Part model, mm, in its own coordinate system. A direction names the side the tool comes from. Round coordinates to 2 decimals unless told otherwise and drop trailing zeros. Loops run counter-clockwise (first coordinate to the right, second up) from the corner with the lowest first, then second, coordinate; pieces in that order, holes last. Notation, with made-up numbers: M 9.5,55.5 L 50.5,55.5 A35 cw 50.5,93.5 Z; hole C 1.5,23 d11. An arc over 180 degrees is marked long. Write each question's results on one line, items separated by ' | '.
from build123d import *

# Parameters (mm, degrees)
SKETCH2_W               = 177.8
SKETCH2_H               = 203.2
BOSS_EXTRUDE1_DEPTH     = 3.175
SKETCH3_W               = 177.8
SKETCH3_H               = 3.175
BOSS_EXTRUDE2_DEPTH     = 127
FILLET1_R               = 3.175
FILLET2_R               = 6.35
CUT_EXTRUDE1_DEPTH      = 255.673793803
CUT_EXTRUDE1_DEPTH_BACK = 255.673793803
FILLET4_R               = 3.175
SKETCH6_R               = 2.54
SKETCH6_R_2             = 2.15
CUT_EXTRUDE2_DEPTH      = 255.673793803
SKETCH7_R               = 4.7625
CUT_EXTRUDE3_DEPTH      = 186.350397895
CONVERT_SOLID1_START    = -88.9
CONVERT_SOLID1_DEPTH    = 177.8


# Read off the part's stored shape, not the designer's step: Convert-Solid1
with BuildPart() as part:
    # Sketch2 → Boss-Extrude1 (new body)
    with BuildSketch(Plane.XY):
        Rectangle(SKETCH2_W, SKETCH2_H)
    extrude(amount=BOSS_EXTRUDE1_DEPTH)

    # Sketch3 → Boss-Extrude2 (add)
    with BuildSketch(Plane.XY.offset(3.175)):
        with Locations((0, -100.0125)):
            Rectangle(SKETCH3_W, SKETCH3_H)
    extrude(amount=BOSS_EXTRUDE2_DEPTH)

    # Fillet1
    fillet1_edges = [part.edges().sort_by_distance(p)[0] for p in [
        (0, -98.425, 3.175),
        (0, -101.6, 0),
    ]]
    fillet(fillet1_edges, radius=FILLET1_R)

    # Fillet2
    fillet2_edges = [part.edges().sort_by_distance(p)[0] for p in [
        (-88.9, -100.0125, 130.175),
        (88.9, -100.0125, 130.175),
        (-88.9, 101.6, 1.5875),
        (88.9, 101.6, 1.5875),
    ]]
    fillet(fillet2_edges, radius=FILLET2_R)

    # Sketch5 → Cut-Extrude1 (cut, two sides: drawn at the far end of the back side and taken through both)
    with BuildSketch(Plane(origin=(0, -98.425, 0), x_dir=(1, 0, 0), z_dir=(0, 1, 0)).offset(-CUT_EXTRUDE1_DEPTH_BACK)):
        Polygon((-485.781273778, -76.2), (-88.9, -76.2), (6.35, -76.2), (6.35, -101.6), (0, -101.6), (0, -130.175), (0, -527.056273778), (-539.971017798, -1108.855450333), (-1025.752291576, -657.999176556), align=None)
    extrude(amount=CUT_EXTRUDE1_DEPTH + CUT_EXTRUDE1_DEPTH_BACK, mode=Mode.SUBTRACT)

    # Fillet4
    fillet4_edges = [part.edges().sort_by_distance(p)[0] for p in [
        (6.35, -100.0125, 101.6),
        (-88.9, -100.0125, 76.2),
        (0, -100.0125, 130.175),
        (0, -100.0125, 101.6),
        (6.35, -100.0125, 76.2),
    ]]
    fillet(fillet4_edges, radius=FILLET4_R - 0.0001)  # a hair under: the kernel refuses the full size

    # Sketch6 → Cut-Extrude2 (cut, through all)
    with BuildSketch(Plane(origin=(0, -98.425, 0), x_dir=(1, 0, 0), z_dir=(0, 1, 0))):
        with Locations(Location((74.6125, -119.0625, 0), (0, 0, 270))):
            Circle(SKETCH6_R)
        with Locations(Location((14.2875, -119.0625, 0), (0, 0, 270))):
            Circle(SKETCH6_R)
        with Locations(Location((14.2875, -58.7375, 0), (0, 0, 270))):
            Circle(SKETCH6_R)
        with Locations(Location((74.6125, -58.7375, 0), (0, 0, 270))):
            Circle(SKETCH6_R)
        with Locations(Location((-29.05, -49.140037229, 0), (0, 0, 270))):
            Circle(SKETCH6_R_2)
        with Locations(Location((-59.05, -49.140037229, 0), (0, 0, 270))):
            Circle(SKETCH6_R_2)
        with Locations(Location((-29.05, -19.440037229, 0), (0, 0, 270))):
            Circle(SKETCH6_R_2)
        with Locations(Location((-59.05, -19.440037229, 0), (0, 0, 270))):
            Circle(SKETCH6_R_2)
    extrude(amount=-CUT_EXTRUDE2_DEPTH, mode=Mode.SUBTRACT)

    # Sketch7 → Cut-Extrude3 (cut, through all)
    with BuildSketch(Plane.XY.offset(3.175)):
        with Locations((-57.15, 82.55)):
            Circle(SKETCH7_R)
        with Locations((57.15, 82.55)):
            Circle(SKETCH7_R)
        with Locations((12.7, -63.5)):
            Circle(SKETCH7_R)
    extrude(amount=-CUT_EXTRUDE3_DEPTH, mode=Mode.SUBTRACT)

    # Convert-Solid1 outline → Convert-Solid1 (cut)
    with BuildSketch(Plane.YZ.offset(CONVERT_SOLID1_START)):
        with BuildLine():
            ThreePointArc((-95.25, 1.5875), (-98.617596045, 2.982403955), (-100.0125, 6.35))
            Line((-100.0125, 6.35), (-100.0125, 130.175))
            Line((-100.0125, 130.175), (-101.6, 130.175))
            Line((-101.6, 130.175), (-101.6, 3.175))
            ThreePointArc((-101.6, 3.175), (-100.67006403, 0.92993597), (-98.425, 0))
            Line((-98.425, 0), (101.6, 0))
            Line((101.6, 0), (101.6, 1.5875))
            Line((101.6, 1.5875), (-95.25, 1.5875))
        make_face()
    extrude(amount=CONVERT_SOLID1_DEPTH, mode=Mode.SUBTRACT)


solid = part.part
Item 1: Two-plate mould, pull along Z, no slides. Class faces 3 (the flat face through (-1, 5, 1.588)), 4 (the cylindrical face through (77.13, -99.21, 118.73)), 5 (the cylindrical face through (86.99, -99.208, 128.364)): +Z half, -Z half, draft (parallel to the pull), parting line (faces both ways), or undercut.
Filled sheet:
face 3: -Z half | face 4: undercut | face 5: +Z half
Item 2: Wall check: L1, parallel to Z at x = -29, y = -99; L2, parallel to Y at x = 14.5, z = 78 (1 decimal); L3, parallel to Z at x = 68, y = 45 (1 decimal). Give the ranges that are in metal, low to high.
Filled sheet:
L1: 3.41 to 17.29, 21.59 to 46.99, 51.29 to 76.2 | L2: -100 to -98.4 | L3: 1.6 to 3.2
Item 3: Drop flat-ended pins along their axis: P1, Ø4, axis at x = -29.05, z = 19.44, coming from the -Y side; P2, Ø11, axis at x = 57.15, y = 82.55, coming from the -Z side; P3, Ø2, axis at x = 29, z = 43, coming from the +Y side (3 decimals); P4, Ø0.8, axis at x = -28.5, y = -99, coming from the +Z side. Give the stop position or say it passes through.
Filled sheet:
P1: through | P2: z = 1.59 | P3: y = -98.425 | P4: z = 76.2
Item 4: Band-saw the part on D-D on z = 11. Give the cut face in (x, y) (1 decimal).
Filled sheet:
outline: M -88.9,-100 L 88.9,-100 L 88.9,-98.4 L -88.9,-98.4 Z
Item 5: Which spindle directions (+Z, -Z, +X, -X, +Y, -Y) get a long thin tool onto all of the face, cutting with end or side? Do faces 1 (the flat face through (19, -98.425, 54)), 2 (the cylindrical face through (12.08, -58.78, 2.39)). Say none if no direction does.
Filled sheet:
face 1: +Z, +X, -X, +Y | face 2: +Z, -Z
Item 6: Band-saw the part on B-B on y = 82.55. Give the cut face in (x, z) (1 decimal).
Filled sheet:
outline: M -88.9,1.6 L -61.9,1.6 L -61.9,3.2 L -88.9,3.2 Z; M -52.4,1.6 L 52.4,1.6 L 52.4,3.2 L -52.4,3.2 Z; M 61.9,1.6 L 88.9,1.6 L 88.9,3.2 L 61.9,3.2 Z
